Could you check a few things on this model? Use its own coordinates, in mm. Face numbers are marked on the shaded views. A direction names the side the tool comes from. Round coordinates to 2 decimals unless told otherwise and drop trailing zeros. Loops run counter-clockwise (first coordinate to the right, second up) from the corner with the lowest first, then second, coordinate; pieces in that order, holes last. Notation, with made-up numbers: (78.5, -30) -> (110.5, -30) arc R26 ccw to (110.5, 6) -> close; hole circle Ø8 at (-6.75, 76.25). An arc over 180 degrees is marked (long way). One line per item, written item: value.
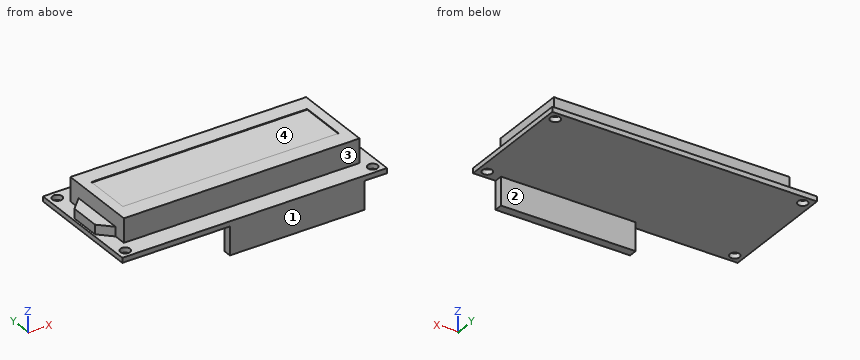
```python
from build123d import *

# Parameters (mm, degrees)
F0_W        = 71.25
F0_H        = 24.4
F0_W_2      = 65.25
F0_H_2      = 14.4
F1_DEPTH    = 7
F2_DEPTH    = 7.2
F3_W        = 17.4
F3_H        = 2.85
F4_DEPTH    = 3.75
F5_T4_DEPTH = 23.4234639037
F5_T9_DEPTH = 23.4234639037
F6_W        = 80
F6_H        = 36.25
F6_R        = 1.5
F7_DEPTH    = 1.5
F8_W        = 40.7
F8_H        = 2.5
F9_DEPTH    = 8.5


# Not quite as in the source:
# - a fillet or chamfer that OpenCascade refuses, or shapes differently, is made with other operations: its cross-section is extruded or revolved along the edge and cut away or added


with BuildPart() as f1:
    # F0 (on Top) → F1 (new body)
    with BuildSketch(Plane.XY):
        Rectangle(F0_W, F0_H)
        Rectangle(F0_W_2, F0_H_2, mode=Mode.SUBTRACT)
        Rectangle(F0_W_2, F0_H_2)
    extrude(amount=F1_DEPTH)

    # F0 (on Top) → F2 (join)
    with BuildSketch(Plane.XY):
        Rectangle(F0_W, F0_H)
        Rectangle(F0_W_2, F0_H_2, mode=Mode.SUBTRACT)
    extrude(amount=F2_DEPTH)

    # F3 (on face) → F4 (join)
    with BuildSketch(Plane(origin=(-35.625, 0, 0), x_dir=(0, -1, 0), z_dir=(-1, 0, 0))):
        with Locations((0, 1.425)):
            Rectangle(F3_W, F3_H)
    extrude(amount=F4_DEPTH)

    # F5: chamfer of 4 on 2 edges, made by hand


with BuildPart() as f5_tool2:
    # F5_s3 → F5_t4 (new body)
    with BuildSketch(Plane.XY.offset(-10.2867319519)):
        Polygon((-35.375, -8.7), (-39.375, -4.7), (-39.375, -8.7), align=None)
    extrude(amount=F5_T4_DEPTH)

    split(bisect_by=Plane.YZ.offset(-35.625), keep=Keep.BOTTOM)


with BuildPart() as f1_1:
    add(f1.part)

    # F5_t1: cut F5_tool2
    add(f5_tool2.part, mode=Mode.SUBTRACT)


with BuildPart() as f5_tool7:
    # F5_s8 → F5_t9 (new body)
    with BuildSketch(Plane.XY.offset(13.1367319519)):
        Polygon((-35.375, 8.7), (-39.375, 4.7), (-39.375, 8.7), align=None)
    extrude(amount=-F5_T9_DEPTH)

    split(bisect_by=Plane.YZ.offset(-35.625), keep=Keep.BOTTOM)


with BuildPart() as f1_2:
    add(f1_1.part)

    # F5_t6: cut F5_tool7
    add(f5_tool7.part, mode=Mode.SUBTRACT)

    # F6 (on Top) → F7 (join)
    with BuildSketch(Plane.XY):
        Rectangle(F6_W, F6_H)
        with Locations((-37.4, -15.525)):
            Circle(F6_R, mode=Mode.SUBTRACT)
        with Locations((37.4, -15.525)):
            Circle(F6_R, mode=Mode.SUBTRACT)
        with Locations((-37.4, 15.525)):
            Circle(F6_R, mode=Mode.SUBTRACT)
        with Locations((37.4, 15.525)):
            Circle(F6_R, mode=Mode.SUBTRACT)
    extrude(amount=-F7_DEPTH)

    # F8 (on face) → F9 (join)
    with BuildSketch(Plane(origin=(0, 0, -1.5), x_dir=(1, 0, 0), z_dir=(0, 0, -1))):
        with Locations((12.85, 16.875)):
            Rectangle(F8_W, F8_H)
    extrude(amount=F9_DEPTH)


solid = f1_2.part
```
(1) Imagine slicing it at D-D on x = -37.4. Write out the boundary of the cut face in (y, z) (3 decimals).
Results below:
outline: (-18.125, -1.5) -> (-17.025, -1.5) -> (-17.025, 0) -> (-18.125, 0) -> close; (-14.025, -1.5) -> (14.025, -1.5) -> (14.025, 0) -> (6.675, 0) -> (6.675, 2.85) -> (-6.675, 2.85) -> (-6.675, 0) -> (-14.025, 0) -> close; (17.025, -1.5) -> (18.125, -1.5) -> (18.125, 0) -> (17.025, 0) -> close
(2) Imagine slicing it at A-A on x = 37.4. Write out the boundary of the cut face in (y, z) (3 decimals), then the cut area to 3 significant figures.
Results below:
outline: (-18.125, -1.5) -> (-17.025, -1.5) -> (-17.025, 0) -> (-18.125, 0) -> close; (-14.025, -1.5) -> (14.025, -1.5) -> (14.025, 0) -> (-14.025, 0) -> close; (17.025, -1.5) -> (18.125, -1.5) -> (18.125, 0) -> (17.025, 0) -> close
area: 45.4 mm²
(3) For pin 1 Ø8 at (x, y) = (-1, 13) entering from -Z; pin 2 Ø1.2 at (y, z) = (-17, -5.5) entering from +X; pin 3 Ø4 at (x, y) = (14.5, 0.5) entering from +Z, each with a flat end and sliding along its axis, tell me the tip position at first contact or that it passes through.
Results below:
pin 1: stops at z = -1.5
pin 2: stops at x = 33.2
pin 3: stops at z = 7
(4) Imagine slicing it at C-C on x = -3.5. Write out the boundary of the cut face in (y, z) (3 decimals).
Results below:
outline: (-18.125, -10) -> (-15.625, -10) -> (-15.625, -1.5) -> (18.125, -1.5) -> (18.125, 0) -> (12.2, 0) -> (12.2, 7.2) -> (7.2, 7.2) -> (7.2, 7) -> (-7.2, 7) -> (-7.2, 7.2) -> (-12.2, 7.2) -> (-12.2, 0) -> (-18.125, 0) -> close
(5) Imagine slicing it at B-B on y = 11. Write out the boundary of the cut face in (x, z) (3 decimals).
Results below:
outline: (-40, -1.5) -> (40, -1.5) -> (40, 0) -> (35.625, 0) -> (35.625, 7.2) -> (-35.625, 7.2) -> (-35.625, 0) -> (-40, 0) -> close
(6) Please list where these lines run through material, in increasing order: L1, parallel to Y at x = 37.4, z = -0.9 (3 decimals); L2, parallel to Y at x = 2.5, z = -6 (3 decimals); L3, parallel to X at y = 7.5, z = 3.5 (3 decimals).
Results below:
L1: y = -18.125 to -17.025, -14.025 to 14.025, 17.025 to 18.125
L2: y = -18.125 to -15.625
L3: x = -35.625 to 35.625
(7) On a 3-axis mill with a long thin cutter (end or side, diameter ignored), from which of +Z, -Z, +X, -X, +Y, -Y can I reach the whole of each face in a straight line? I mean the marked faces 1, 2, 3 and 4. Say none if no direction works.
Results below:
face 1: +Z, -Z, +X, -X, -Y
face 2: -Z, +X, -X, +Y
face 3: +Z, +X, -X, -Y
face 4: +Z
